Geometry check sheet. Reference: drawing and pictorial views, mm from the part's lowest x, y, z. Coordinates: 2 decimals unless noted, no trailing zeros. Loops run counter-clockwise (first coordinate to the right, second up) from the corner with the lowest first, then second, coordinate; pieces in that order, holes last. Notation, with made-up numbers: (-23.5, 41) - (-11.5, 41) arc R14 cw to (-11.5, 64) - close; hole circle Ø8 at (-10.75, -17.5). An arc over 180 degrees is marked (long way). One line per item, written item: value.
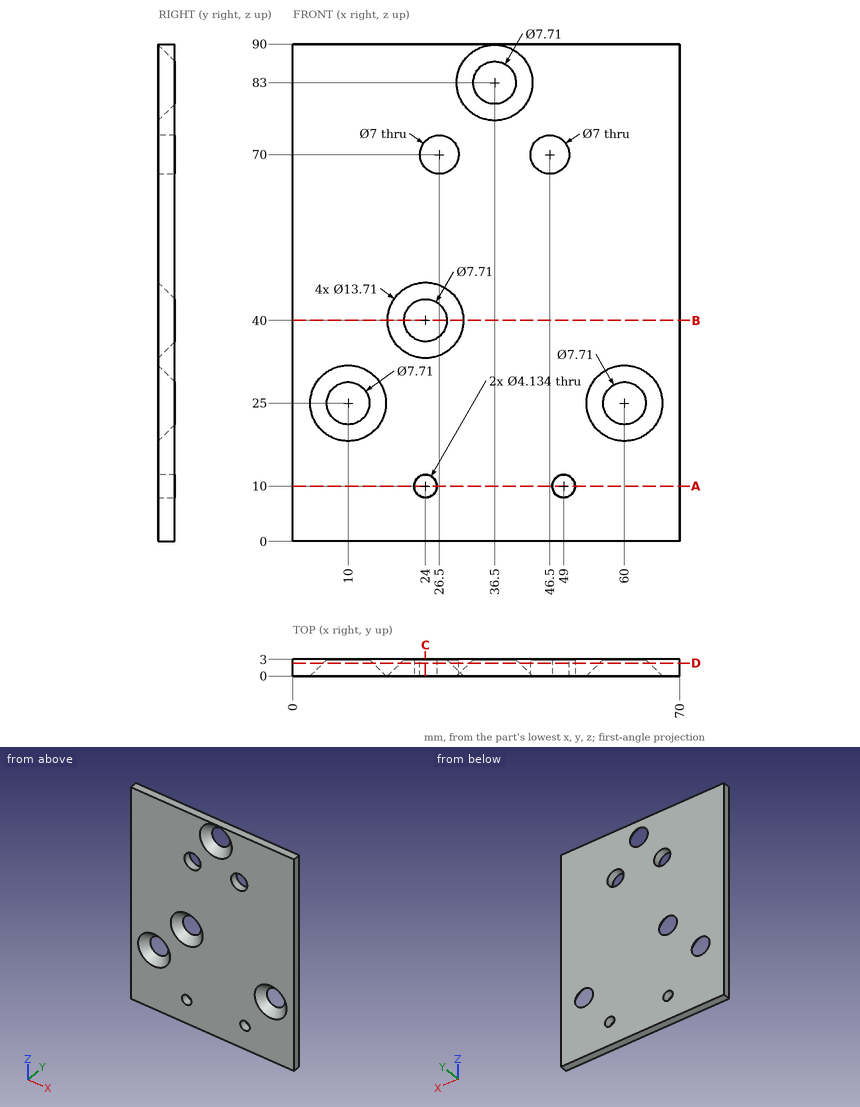
(1) Cross-section at D-D on y = 2.35. State how many separate pieces and enclosed holes the cut face has, and give its area (3 significant figures).
Reply:
separate pieces: 1
enclosed holes: 8
area: 5,940 mm2
(2) Cross-section at C-C on x = 24. Record the cut outline in (y, z) (3 decimals).
Reply:
outline: (0, 0) - (3, 0) - (3, 7.933) - (0, 7.933) - close; (0, 12.067) - (3, 12.067) - (3, 36.145) - (0, 33.145) - close; (0, 46.855) - (3, 43.855) - (3, 67.551) - (0, 67.551) - close; (0, 72.449) - (3, 72.449) - (3, 90) - (0, 90) - close
(3) Cross-section at A-A on z = 10. Record the cut outline in (x, y), and give its area (3 significant figures).
Reply:
outline: (0, 0) - (21.93, 0) - (21.93, 3) - (0, 3) - close; (26.07, 0) - (46.93, 0) - (46.93, 3) - (26.07, 3) - close; (51.07, 0) - (70, 0) - (70, 3) - (51.07, 3) - close
area: 185 mm2
(4) Cross-section at B-B on z = 40. Record the cut outline in (x, y) (3 decimals), and give its area (3 significant figures).
Reply:
outline: (0, 0) - (17.145, 0) - (20.145, 3) - (0, 3) - close; (27.855, 3) - (30.855, 0) - (70, 0) - (70, 3) - close
area: 178 mm2
(5) Material ranges on probe 1 along X at (y, z) = (1.35, 10); probe 2 along X at (y, z) = (2.3, 70); probe 3 along Z at (x, y) = (24, 1.3) (3 decimals), recorded low to high. Write a range as from..to.
Reply:
probe 1: 0..21.93, 26.07..46.93, 51.07..70
probe 2: 0..23, 30..43, 50..70
probe 3: 0..7.933, 12.067..34.445, 45.555..67.551, 72.449..90
(6) Go/stop test with a flat-tipped pin: pin 1 Ø3.5 at (x, z) = (49, 10) entering from +Y. Record where the tip stops, or that it passes through.
Reply:
pin 1: through
